The model under review builds one solid part; all positions refer to its coordinate system, in mm. A direction names the side the tool comes from. Coordinates: 2 decimals unless noted, no trailing zeros. Loops run counter-clockwise (first coordinate to the right, second up) from the corner with the lowest first, then second, coordinate; pieces in that order, holes last. Notation, with made-up numbers: M 75.25,64.5 L 120.25,64.5 A23 cw 120.25,98.5 Z; hole C -30,64 d1. An arc over 180 degrees is marked long. One line per item, written item: value.
```python
from build123d import *

# Parameters (mm, degrees)
SKETCH_1_R               = 7.5
EXTRUDE_1_DEPTH          = 1
EXTRUDE_2_DEPTH          = 7
SKETCH_3_R               = 7.5
EXTRUDE_3_DEPTH          = 9
CUT_EXTRUDE_1_REACH      = 22.037
SKETCH_4_R               = 3
CUT_EXTRUDE_2_REACH      = 22.037
CUT_EXTRUDE_2_END_RADIUS = 7.5
SKETCH_5_R               = 2


with BuildPart() as part:
    # 草图1 → 凸台-拉伸1 (new body)
    with BuildSketch(Plane(origin=(0, 0, 0), x_dir=(1, 0, 0), z_dir=(0, 1, 0))):
        with Locations(Location((0, 0, 0), (0, 0, 270))):
            Circle(SKETCH_1_R)
    extrude(amount=EXTRUDE_1_DEPTH)

    # 草图2 → 凸台-拉伸2 (add)
    with BuildSketch(Plane(origin=(0, 1, 0), x_dir=(1, 0, 0), z_dir=(0, 1, 0))):
        with BuildLine():
            Line((-0.35, 6.055518957), (-0.35, 6.455518957))
            ThreePointArc((-0.35, 6.455518957), (-1.011348816, 6.385405122), (-1.661995284, 6.247719318))
            Line((-1.661995284, 6.247719318), (-1.538388487, 5.867296711))
            Line((-1.538388487, 5.867296711), (-2.204128048, 5.650984815))
            Line((-2.204128048, 5.650984815), (-2.327734846, 6.031407422))
            ThreePointArc((-2.327734846, 6.031407422), (-2.935048581, 5.760357179), (-3.511302891, 5.428349382))
            Line((-3.511302891, 5.428349382), (-3.27618879, 5.104742584))
            Line((-3.27618879, 5.104742584), (-3.842500686, 4.693292907))
            Line((-3.842500686, 4.693292907), (-4.077614787, 5.016899705))
            ThreePointArc((-4.077614787, 5.016899705), (-4.57144534, 4.57144534), (-5.016899705, 4.077614787))
            Line((-5.016899705, 4.077614787), (-4.693292907, 3.842500686))
            Line((-4.693292907, 3.842500686), (-5.104742584, 3.27618879))
            Line((-5.104742584, 3.27618879), (-5.428349382, 3.511302891))
            ThreePointArc((-5.428349382, 3.511302891), (-5.760357179, 2.935048581), (-6.031407422, 2.327734846))
            Line((-6.031407422, 2.327734846), (-5.650984815, 2.204128048))
            Line((-5.650984815, 2.204128048), (-5.867296711, 1.538388487))
            Line((-5.867296711, 1.538388487), (-6.247719318, 1.661995284))
            ThreePointArc((-6.247719318, 1.661995284), (-6.385405122, 1.011348816), (-6.455518957, 0.35))
            Line((-6.455518957, 0.35), (-6.055518957, 0.35))
            Line((-6.055518957, 0.35), (-6.055518957, -0.35))
            Line((-6.055518957, -0.35), (-6.455518957, -0.35))
            ThreePointArc((-6.455518957, -0.35), (-6.385405122, -1.011348816), (-6.247719318, -1.661995284))
            Line((-6.247719318, -1.661995284), (-5.867296711, -1.538388487))
            Line((-5.867296711, -1.538388487), (-5.650984815, -2.204128048))
            Line((-5.650984815, -2.204128048), (-6.031407422, -2.327734846))
            ThreePointArc((-6.031407422, -2.327734846), (-5.760357179, -2.935048581), (-5.428349382, -3.511302891))
            Line((-5.428349382, -3.511302891), (-5.104742584, -3.27618879))
            Line((-5.104742584, -3.27618879), (-4.693292907, -3.842500686))
            Line((-4.693292907, -3.842500686), (-5.016899705, -4.077614787))
            ThreePointArc((-5.016899705, -4.077614787), (-4.57144534, -4.57144534), (-4.077614787, -5.016899705))
            Line((-4.077614787, -5.016899705), (-3.842500686, -4.693292907))
            Line((-3.842500686, -4.693292907), (-3.27618879, -5.104742584))
            Line((-3.27618879, -5.104742584), (-3.511302891, -5.428349382))
            ThreePointArc((-3.511302891, -5.428349382), (-2.935048581, -5.760357179), (-2.327734846, -6.031407422))
            Line((-2.327734846, -6.031407422), (-2.204128048, -5.650984815))
            Line((-2.204128048, -5.650984815), (-1.538388487, -5.867296711))
            Line((-1.538388487, -5.867296711), (-1.661995284, -6.247719318))
            ThreePointArc((-1.661995284, -6.247719318), (-1.011348816, -6.385405122), (-0.35, -6.455518957))
            Line((-0.35, -6.455518957), (-0.35, -6.055518957))
            Line((-0.35, -6.055518957), (0.35, -6.055518957))
            Line((0.35, -6.055518957), (0.35, -6.455518957))
            ThreePointArc((0.35, -6.455518957), (1.011348816, -6.385405122), (1.661995284, -6.247719318))
            Line((1.661995284, -6.247719318), (1.538388487, -5.867296711))
            Line((1.538388487, -5.867296711), (2.204128048, -5.650984815))
            Line((2.204128048, -5.650984815), (2.327734846, -6.031407422))
            ThreePointArc((2.327734846, -6.031407422), (2.935048581, -5.760357179), (3.511302891, -5.428349382))
            Line((3.511302891, -5.428349382), (3.27618879, -5.104742584))
            Line((3.27618879, -5.104742584), (3.842500686, -4.693292907))
            Line((3.842500686, -4.693292907), (4.077614787, -5.016899705))
            ThreePointArc((4.077614787, -5.016899705), (4.57144534, -4.57144534), (5.016899705, -4.077614787))
            Line((5.016899705, -4.077614787), (4.693292907, -3.842500686))
            Line((4.693292907, -3.842500686), (5.104742584, -3.27618879))
            Line((5.104742584, -3.27618879), (5.428349382, -3.511302891))
            ThreePointArc((5.428349382, -3.511302891), (5.760357179, -2.935048581), (6.031407422, -2.327734846))
            Line((6.031407422, -2.327734846), (5.650984815, -2.204128048))
            Line((5.650984815, -2.204128048), (5.867296711, -1.538388487))
            Line((5.867296711, -1.538388487), (6.247719318, -1.661995284))
            ThreePointArc((6.247719318, -1.661995284), (6.385405122, -1.011348816), (6.455518957, -0.35))
            Line((6.455518957, -0.35), (6.055518957, -0.35))
            Line((6.055518957, -0.35), (6.055518957, 0.35))
            Line((6.055518957, 0.35), (6.455518957, 0.35))
            ThreePointArc((6.455518957, 0.35), (6.385405122, 1.011348816), (6.247719318, 1.661995284))
            Line((6.247719318, 1.661995284), (5.867296711, 1.538388487))
            Line((5.867296711, 1.538388487), (5.650984815, 2.204128048))
            Line((5.650984815, 2.204128048), (6.031407422, 2.327734846))
            ThreePointArc((6.031407422, 2.327734846), (5.760357179, 2.935048581), (5.428349382, 3.511302891))
            Line((5.428349382, 3.511302891), (5.104742584, 3.27618879))
            Line((5.104742584, 3.27618879), (4.693292907, 3.842500686))
            Line((4.693292907, 3.842500686), (5.016899705, 4.077614787))
            ThreePointArc((5.016899705, 4.077614787), (4.57144534, 4.57144534), (4.077614787, 5.016899705))
            Line((4.077614787, 5.016899705), (3.842500686, 4.693292907))
            Line((3.842500686, 4.693292907), (3.27618879, 5.104742584))
            Line((3.27618879, 5.104742584), (3.511302891, 5.428349382))
            ThreePointArc((3.511302891, 5.428349382), (2.935048581, 5.760357179), (2.327734846, 6.031407422))
            Line((2.327734846, 6.031407422), (2.204128048, 5.650984815))
            Line((2.204128048, 5.650984815), (1.538388487, 5.867296711))
            Line((1.538388487, 5.867296711), (1.661995284, 6.247719318))
            ThreePointArc((1.661995284, 6.247719318), (1.011348816, 6.385405122), (0.35, 6.455518957))
            Line((0.35, 6.455518957), (0.35, 6.055518957))
            Line((0.35, 6.055518957), (-0.35, 6.055518957))
        make_face()
    extrude(amount=EXTRUDE_2_DEPTH)

    # 草图3 → 凸台-拉伸3 (add)
    with BuildSketch(Plane(origin=(0, 8, 0), x_dir=(1, 0, 0), z_dir=(0, 1, 0))):
        with Locations(Location((0, 0, 0), (0, 0, 270))):
            Circle(SKETCH_3_R)
    extrude(amount=EXTRUDE_3_DEPTH)

    # 草图4 → 切除-拉伸1 (cut, up to next)
    with BuildSketch(Plane(origin=(0, 17, 0), x_dir=(1, 0, 0), z_dir=(0, 1, 0)), mode=Mode.PRIVATE) as cut_extrude_1_sk1:
        with Locations(Location((0, 0, 0), (0, 0, 270))):
            Circle(SKETCH_4_R)
    cut_extrude_1_tool1 = extrude(cut_extrude_1_sk1.sketch, amount=-CUT_EXTRUDE_1_REACH, mode=Mode.PRIVATE) & part.part
    add(cut_extrude_1_tool1.solids().sort_by_distance((0, 17, 0))[0], mode=Mode.SUBTRACT)

    # 切除-拉伸2: up to this cylinder (the profile starts inside it)
    cut_extrude_2_end = Plane(origin=(0, 12.5, 0), z_dir=(0, -1, 0)) * Cylinder(CUT_EXTRUDE_2_END_RADIUS, 60.074, mode=Mode.PRIVATE)
    # 草图5 → 切除-拉伸2 (cut, up to the surface)
    with BuildSketch(Plane(origin=(0, 0, 0), x_dir=(0, 0, -1), z_dir=(1, 0, 0)), mode=Mode.PRIVATE) as cut_extrude_2_sk1:
        with Locations((0, 12.5)):
            Circle(SKETCH_5_R)
    cut_extrude_2_tool1 = extrude(cut_extrude_2_sk1.sketch, amount=-CUT_EXTRUDE_2_REACH, mode=Mode.PRIVATE) & cut_extrude_2_end
    add(cut_extrude_2_tool1.solids().sort_by_distance((0, 12.5, 0))[0], mode=Mode.SUBTRACT)


solid = part.part
```
(1) To check wall thickness, follow L1, parallel to X at y = 4.75, z = 0; L2, parallel to Y at x = -3, z = 6.5; L3, parallel to Z at x = -1.5, y = 8.25. State the ranges of each line that lie inside material, in increasing order. Write a range as [from, to].
Checks:
L1: [-6.06, -3], [3, 6.06]
L2: [0, 1], [8, 17]
L3: [-7.35, -2.6], [2.6, 7.35]
(2) Draft analysis for pull direction Z (two halves, no side actions). For faces 6 (the face through (2.927, 4.451, 5.765)), 7 (the face through (3, 9, 0)), 8 (the face through (2.94, 4.45, -5.76)), state which applies: pulls with the +Z half, pulls with the -Z half, needs draft (parallel to the pull), parting line crosses it, or undercut.
Checks:
face 6: pulls with the +Z half
face 7: undercut
face 8: pulls with the -Z half
(3) Add section A-A on x = 0. State the section outline as (y, z) points.
Checks:
outline: M 0,-7.5 L 1,-7.5 L 1,-6.06 L 8,-6.06 L 8,-7.5 L 17,-7.5 L 17,-3 L 0,-3 Z; M 0,3 L 17,3 L 17,7.5 L 8,7.5 L 8,6.06 L 1,6.06 L 1,7.5 L 0,7.5 Z
(4) Tool access review of faces 1 (the face through (1.002, 4.451, 6.387)), 2 (the face through (6, 1, 2)), 3 (the face through (-6.384, 4.451, -1.021)), 4 (the face through (-5.765, 4.451, 2.927)), 5 (the face through (6.387, 4.451, -1.002)): name each direction out of +Z, -Z, +X, -X, +Y, -Y from which nothing blocks a thin tool from reaching the whole face with its end or side.
Checks:
face 1: +Z, +X
face 2: none
face 3: -Z, -X
face 4: +Z, -X
face 5: -Z, +X
(5) Insertion check: pin 1 Ø0.8 at (y, z) = (5.5, 0) entering from +X; pin 2 Ø1 at (y, z) = (14, -2) entering from -X; pin 3 Ø4 at (x, y) = (4, 14.5) entering from -Z. Each pin has a flat end and moves straight along its axis. Give the tip position at first contact, or say it passes through.
Checks:
pin 1: x = 6.46
pin 2: x = -7.35
pin 3: z = -7.23
(6) Add section C-C on y = 15. State the section outline as (x, z) points, then the cut area to 3 significant figures.
Checks:
outline: C 0,0 d15; hole C 0,0 d6
area: 148 mm^2
(7) Add section B-B on z = 0. State the section outline as (x, y) points, then the cut area to 3 significant figures.
Checks:
outline: M -7.5,0 L -3,0 L -3,10.5 L -7.5,10.5 L -7.5,8 L -6.06,8 L -6.06,1 L -7.5,1 Z; M -7.5,14.5 L -3,14.5 L -3,17 L -7.5,17 Z; M 3,0 L 7.5,0 L 7.5,1 L 6.06,1 L 6.06,8 L 7.5,8 L 7.5,17 L 3,17 Z
area: 115 mm^2
